The model under review builds one solid part; all positions refer to its coordinate system, in mm. Round coordinates to 2 decimals unless told otherwise and drop trailing zeros. Answer as CSV lines item,"result".
from build123d import *

# Parameters (mm, degrees)
F0_R     = 1.85
F0_R_2   = 4
F2_DEPTH = 3


with BuildPart() as f2:
    # F0 (on Top) → F2 (new body)
    with BuildSketch(Plane.XY):
        with BuildLine():
            Line((91, 96), (5, 96))
            ThreePointArc((5, 96), (1.4644660941, 94.5355339059), (0, 91))
            Line((0, 91), (0, 5))
            ThreePointArc((0, 5), (1.4644660941, 1.4644660941), (5, 0))
            Line((5, 0), (91, 0))
            ThreePointArc((91, 0), (94.5355339059, 1.4644660941), (96, 5))
            Line((96, 5), (96, 91))
            ThreePointArc((96, 91), (94.5355339059, 94.5355339059), (91, 96))
        make_face()
        with Locations((10.3431457505, 10.3431457505)):
            Circle(F0_R, mode=Mode.SUBTRACT)
        with Locations((16, 8)):
            Circle(F0_R, mode=Mode.SUBTRACT)
        with Locations((21.6568542495, 10.3431457505)):
            Circle(F0_R, mode=Mode.SUBTRACT)
        with Locations((8, 16)):
            Circle(F0_R, mode=Mode.SUBTRACT)
        with Locations((10.3431457505, 21.6568542495)):
            Circle(F0_R, mode=Mode.SUBTRACT)
        with Locations((16, 16)):
            Circle(F0_R_2, mode=Mode.SUBTRACT)
        with Locations((21.6568542495, 21.6568542495)):
            Circle(F0_R, mode=Mode.SUBTRACT)
        with Locations((42.3431457505, 10.3431457505)):
            Circle(F0_R, mode=Mode.SUBTRACT)
        with Locations((24, 16)):
            Circle(F0_R, mode=Mode.SUBTRACT)
        with Locations((40, 16)):
            Circle(F0_R, mode=Mode.SUBTRACT)
        with Locations((42.3431457505, 21.6568542495)):
            Circle(F0_R, mode=Mode.SUBTRACT)
        with Locations((16, 24)):
            Circle(F0_R, mode=Mode.SUBTRACT)
        with Locations((10.3431457505, 42.3431457505)):
            Circle(F0_R, mode=Mode.SUBTRACT)
        with Locations((16, 40)):
            Circle(F0_R, mode=Mode.SUBTRACT)
        with Locations((21.6568542495, 42.3431457505)):
            Circle(F0_R, mode=Mode.SUBTRACT)
        with Locations((42.3431457505, 42.3431457505)):
            Circle(F0_R, mode=Mode.SUBTRACT)
        with Locations((48, 8)):
            Circle(F0_R, mode=Mode.SUBTRACT)
        with Locations((53.6568542495, 10.3431457505)):
            Circle(F0_R, mode=Mode.SUBTRACT)
        with Locations((48, 16)):
            Circle(F0_R_2, mode=Mode.SUBTRACT)
        with Locations((56, 16)):
            Circle(F0_R, mode=Mode.SUBTRACT)
        with Locations((53.6568542495, 21.6568542495)):
            Circle(F0_R, mode=Mode.SUBTRACT)
        with Locations((74.3431457505, 10.3431457505)):
            Circle(F0_R, mode=Mode.SUBTRACT)
        with Locations((80, 8)):
            Circle(F0_R, mode=Mode.SUBTRACT)
        with Locations((85.6568542495, 10.3431457505)):
            Circle(F0_R, mode=Mode.SUBTRACT)
        with Locations((72, 16)):
            Circle(F0_R, mode=Mode.SUBTRACT)
        with Locations((80, 16)):
            Circle(F0_R_2, mode=Mode.SUBTRACT)
        with Locations((74.3431457505, 21.6568542495)):
            Circle(F0_R, mode=Mode.SUBTRACT)
        with Locations((88, 16)):
            Circle(F0_R, mode=Mode.SUBTRACT)
        with Locations((85.6568542495, 21.6568542495)):
            Circle(F0_R, mode=Mode.SUBTRACT)
        with Locations((48, 24)):
            Circle(F0_R, mode=Mode.SUBTRACT)
        with Locations((48, 40)):
            Circle(F0_R, mode=Mode.SUBTRACT)
        with Locations((53.6568542495, 42.3431457505)):
            Circle(F0_R, mode=Mode.SUBTRACT)
        with Locations((80, 24)):
            Circle(F0_R, mode=Mode.SUBTRACT)
        with Locations((80, 40)):
            Circle(F0_R, mode=Mode.SUBTRACT)
        with Locations((74.3431457505, 42.3431457505)):
            Circle(F0_R, mode=Mode.SUBTRACT)
        with Locations((85.6568542495, 42.3431457505)):
            Circle(F0_R, mode=Mode.SUBTRACT)
        with Locations((8, 48)):
            Circle(F0_R, mode=Mode.SUBTRACT)
        with Locations((10.3431457505, 53.6568542495)):
            Circle(F0_R, mode=Mode.SUBTRACT)
        with Locations((16, 48)):
            Circle(F0_R_2, mode=Mode.SUBTRACT)
        with Locations((21.6568542495, 53.6568542495)):
            Circle(F0_R, mode=Mode.SUBTRACT)
        with Locations((16, 56)):
            Circle(F0_R, mode=Mode.SUBTRACT)
        with Locations((24, 48)):
            Circle(F0_R, mode=Mode.SUBTRACT)
        with Locations((40, 48)):
            Circle(F0_R, mode=Mode.SUBTRACT)
        with Locations((42.3431457505, 53.6568542495)):
            Circle(F0_R, mode=Mode.SUBTRACT)
        with Locations((10.3431457505, 74.3431457505)):
            Circle(F0_R, mode=Mode.SUBTRACT)
        with Locations((8, 80)):
            Circle(F0_R, mode=Mode.SUBTRACT)
        with Locations((16, 72)):
            Circle(F0_R, mode=Mode.SUBTRACT)
        with Locations((21.6568542495, 74.3431457505)):
            Circle(F0_R, mode=Mode.SUBTRACT)
        with Locations((16, 80)):
            Circle(F0_R_2, mode=Mode.SUBTRACT)
        with Locations((10.3431457505, 85.6568542495)):
            Circle(F0_R, mode=Mode.SUBTRACT)
        with Locations((16, 88)):
            Circle(F0_R, mode=Mode.SUBTRACT)
        with Locations((21.6568542495, 85.6568542495)):
            Circle(F0_R, mode=Mode.SUBTRACT)
        with Locations((24, 80)):
            Circle(F0_R, mode=Mode.SUBTRACT)
        with Locations((42.3431457505, 74.3431457505)):
            Circle(F0_R, mode=Mode.SUBTRACT)
        with Locations((40, 80)):
            Circle(F0_R, mode=Mode.SUBTRACT)
        with Locations((42.3431457505, 85.6568542495)):
            Circle(F0_R, mode=Mode.SUBTRACT)
        with Locations((48, 48)):
            Circle(F0_R_2, mode=Mode.SUBTRACT)
        with Locations((53.6568542495, 53.6568542495)):
            Circle(F0_R, mode=Mode.SUBTRACT)
        with Locations((56, 48)):
            Circle(F0_R, mode=Mode.SUBTRACT)
        with Locations((48, 56)):
            Circle(F0_R, mode=Mode.SUBTRACT)
        with Locations((72, 48)):
            Circle(F0_R, mode=Mode.SUBTRACT)
        with Locations((74.3431457505, 53.6568542495)):
            Circle(F0_R, mode=Mode.SUBTRACT)
        with Locations((80, 48)):
            Circle(F0_R_2, mode=Mode.SUBTRACT)
        with Locations((80, 56)):
            Circle(F0_R, mode=Mode.SUBTRACT)
        with Locations((88, 48)):
            Circle(F0_R, mode=Mode.SUBTRACT)
        with Locations((85.6568542495, 53.6568542495)):
            Circle(F0_R, mode=Mode.SUBTRACT)
        with Locations((48, 72)):
            Circle(F0_R, mode=Mode.SUBTRACT)
        with Locations((53.6568542495, 74.3431457505)):
            Circle(F0_R, mode=Mode.SUBTRACT)
        with Locations((48, 80)):
            Circle(F0_R_2, mode=Mode.SUBTRACT)
        with Locations((56, 80)):
            Circle(F0_R, mode=Mode.SUBTRACT)
        with Locations((53.6568542495, 85.6568542495)):
            Circle(F0_R, mode=Mode.SUBTRACT)
        with Locations((48, 88)):
            Circle(F0_R, mode=Mode.SUBTRACT)
        with Locations((74.3431457505, 74.3431457505)):
            Circle(F0_R, mode=Mode.SUBTRACT)
        with Locations((80, 72)):
            Circle(F0_R, mode=Mode.SUBTRACT)
        with Locations((72, 80)):
            Circle(F0_R, mode=Mode.SUBTRACT)
        with Locations((80, 80)):
            Circle(F0_R_2, mode=Mode.SUBTRACT)
        with Locations((85.6568542495, 74.3431457505)):
            Circle(F0_R, mode=Mode.SUBTRACT)
        with Locations((88, 80)):
            Circle(F0_R, mode=Mode.SUBTRACT)
        with Locations((74.3431457505, 85.6568542495)):
            Circle(F0_R, mode=Mode.SUBTRACT)
        with Locations((80, 88)):
            Circle(F0_R, mode=Mode.SUBTRACT)
        with Locations((85.6568542495, 85.6568542495)):
            Circle(F0_R, mode=Mode.SUBTRACT)
    extrude(amount=F2_DEPTH)


solid = f2.part
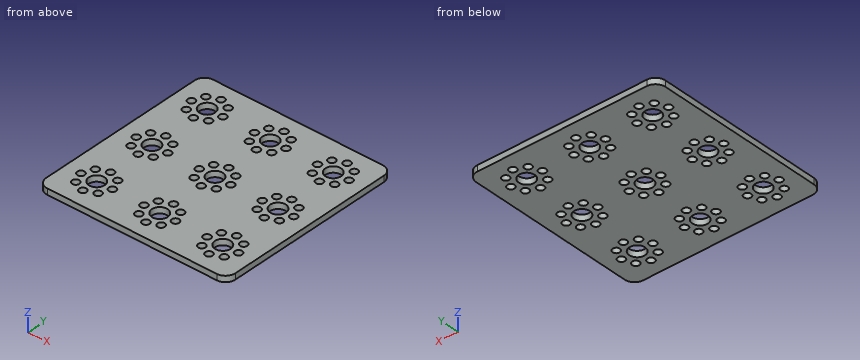
1. Wall thickness on probe 1 along Y at (x, z) = (72, 1.3); probe 2 along X at (y, z) = (50.5, 0.2): over which ranges is each line inside the solid? List them lowest first.
Numbers:
probe 1,"y = 0 to 14.15, 17.85 to 46.15, 49.85 to 78.15, 81.85 to 96"
probe 2,"x = 0 to 12.88, 19.12 to 44.88, 51.12 to 76.88, 83.12 to 96"
2. Take a section at A-A (y = 80). State how many separate pieces and enclosed holes the cut face has, plus the area to 3 significant figures.
Numbers:
separate pieces,"10"
enclosed holes,"0"
area,"149 mm²"
3. Clearance check with a flat-ended pin moving along its axis: pin 1 (2 mm diameter, centred on x = 48, y = 56, fed in from +Z). State where the tip first meets the part, or that it passes through.
Numbers:
pin 1,"passes through"
